```python
from build123d import *

# Parameters (mm, degrees)
F0_W     = 203.2
F0_H     = 101.6
F1_DEPTH = 63.5
F3_DEPTH = 203.2
F4_R     = 2.286


with BuildPart() as f1:
    # F0 (on Top) → F1 (new body)
    with BuildSketch(Plane.XY):
        with Locations((101.6, 50.8)):
            Rectangle(F0_W, F0_H)
    extrude(amount=F1_DEPTH)

    # F2 (on face) → F3 (cut, through all)
    with BuildSketch(Plane.YZ.offset(203.2)):
        Polygon((25.4, 38.1), (0, 63.5), (0, 38.1), align=None)
        Polygon((101.6, 38.1), (101.6, 63.5), (76.2, 38.1), align=None)
    extrude(amount=-F3_DEPTH, mode=Mode.SUBTRACT)

    # F4
    f4_edges = [f1.edges().sort_by_distance(p)[0] for p in [
        (203.2, 50.8, 63.5),
        (203.2, 12.7, 50.8),
        (203.2, 12.7, 38.1),
        (203.2, 0, 19.05),
        (203.2, 50.8, 0),
        (203.2, 101.6, 19.05),
        (203.2, 88.9, 38.1),
        (203.2, 88.9, 50.8),
        (101.6, 0, 38.1),
        (101.6, 0, 63.5),
        (0, 0, 19.05),
        (0, 12.7, 38.1),
        (0, 12.7, 50.8),
        (0, 50.8, 63.5),
        (0, 88.9, 50.8),
        (0, 88.9, 38.1),
        (0, 101.6, 19.05),
        (101.6, 101.6, 38.1),
        (101.6, 101.6, 63.5),
    ]]
    fillet(f4_edges, radius=F4_R)


solid = f1.part
```
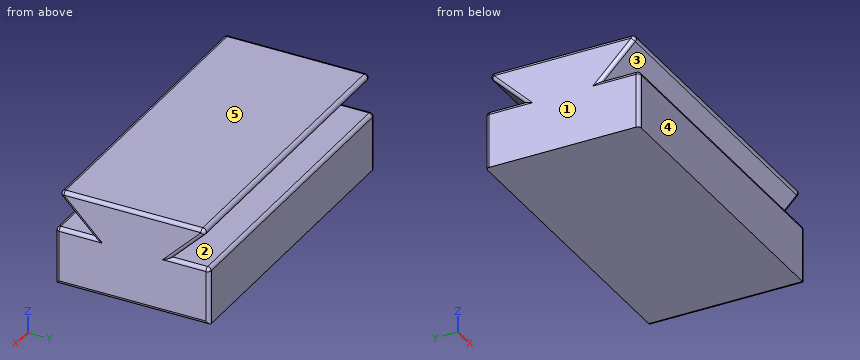
CAD build for the part. Positions are in the model's coordinates, mm. Face numbers are marked on the shaded views. A direction names the side the tool comes from. Give positions to 0.01 mm unless a question says otherwise; leave off trailing zeros. Loops run counter-clockwise (first coordinate to the right, second up) from the corner with the lowest first, then second, coordinate; pieces in that order, holes last. Notation, with made-up numbers: M -14,27 L 31,27 A20 ccw 31,60 Z; hole C 27,87.25 d6. An arc over 180 degrees is marked long. Use one line per item in the form item = value.
Item 1: Two-plate mould, pull along Z, no slides. Class the marked faces 3, 4 and 5: pulls with the +Z half, pulls with the -Z half, needs draft (parallel to the pull), parting line crosses it, or undercut.
Determined:
face_3 = undercut
face_4 = needs draft
face_5 = pulls with the +Z half
Item 2: Slice it at A-A (x = 170). List the corners of the cut face in (y, z).
Determined:
outline = M 0,0 L 101.6,0 L 101.6,35.81 A2.29 ccw 99.31,38.1 L 76.2,38.1 L 97.7,59.6 A2.29 ccw 96.08,63.5 L 5.52,63.5 A2.29 ccw 3.9,59.6 L 25.4,38.1 L 2.29,38.1 A2.29 ccw 0,35.81 Z
Item 3: Which spindle directions (+Z, -Z, +X, -X, +Y, -Y) get a long thin tool onto all of the face, cutting with end or side? Do the marked faces 1 and 2. Say none if no direction does.
Determined:
face_1 = +Z, -Z, -X, +Y, -Y
face_2 = +X, -X, +Y
Item 4: Flat gauge pins, fed straight in: pin 1 (10 mm diameter, centred on x = 175.5, z = 55.5, fed in from +Y); pin 2 (4 mm diameter, centred on x = 33, z = 57, fed in from -Y); pin 3 (1 mm diameter, centred on x = 83.5, z = 42.5, fed in from -Y). Where does each tip first touch, or does it go through?
Determined:
pin_1 = 98.25
pin_2 = 4.5
pin_3 = 20.5
Item 5: Drill centre lines: probe 1 along Z at (x, y) = (14.5, 19.5); probe 2 along Z at (x, y) = (179.5, 21.5); probe 3 along Y at (x, z) = (91, 60.5). Where is each one in solid material? Low to high. Write a range as from..to.
Determined:
probe_1 = 0..38.1, 44..63.5
probe_2 = 0..38.1, 42..63.5
probe_3 = 3.35..98.25
